```python
from build123d import *

# Parameters (mm, degrees)
F0_W     = 40
F0_H     = 10
F1_DEPTH = 5
F2_DEPTH = 92
F3_DEPTH = 50


with BuildPart() as f1:
    # F0 (on Top) → F1 (new body)
    with BuildSketch(Plane.XY):
        with Locations((-1.222661, 7.045219)):
            Rectangle(F0_W, F0_H)
    extrude(amount=F1_DEPTH)

    # F0 (on Top) → F2 (join)
    with BuildSketch(Plane.XY):
        Polygon((-26.222661, 12.045219), (-21.222661, 12.045219), (18.777339, 12.045219), (23.777339, 12.045219), (23.777339, 17.045219), (-26.222661, 17.045219), align=None)
    extrude(amount=F2_DEPTH)

    # F0 (on Top) → F3 (join)
    with BuildSketch(Plane.XY):
        Polygon((-21.222661, 2.045219), (-21.222661, 12.045219), (-26.222661, 12.045219), (-26.222661, -2.954781), (23.777339, -2.954781), (23.777339, 12.045219), (18.777339, 12.045219), (18.777339, 2.045219), align=None)
    extrude(amount=F3_DEPTH)


solid = f1.part
```
Build history of the part. All positions in model axes, mm. A direction names the side the tool comes from. Round coordinates to 2 decimals unless told otherwise and drop trailing zeros. Write each loop counter-clockwise with the first axis right and the second up, starting at its lowest first coordinate (ties: lowest second). Pieces come first, ordered by that corner, then holes.
1) Band-saw the part on C-C, the plane y = 4.5. List the corners of the cut face in (x, z).
2) 3-axis set-ups, long thin cutter, end or side, ignore diameter. For faces 4 (the flat face through (-21.223, 7, 27)), 5 (the flat face through (-26.223, 9, 35)), 6 (the flat face through (-2, 1, 50)): which of +Z, -Z, +X, -X, +Y, -Y reach the whole face in a straight line?
3) Mould opens along Y. For faces 1 (the flat face through (-2, 12.045, 48)), 2 (the flat face through (-2, 7, 0)), 3 (the flat face through (-2, -2.955, 25)) say: +Y half, -Y half, draft (parallel to the pull), parting line (faces both ways), or undercut.
4) Band-saw the part on D-D, the plane z = 55. List the corners of the cut face in (x, y).
5) Band-saw the part on B-B, the plane x = -4. List the corners of the cut face in (y, z), and give its area (3 significant figures).
6) Pin check, flat tips, straight feed: pin 1 (7.5 mm diameter, centred on x = 0, y = 6.5, fed in from +Z); pin 2 (11 mm diameter, centred on x = -9, y = 6.5, fed in from +Z); pin 3 (25 mm diameter, centred on x = 9, z = 67, fed in from -Y). Stop position of each tip, or through.
7) Drill centre lines: probe 1 along Y at (x, z) = (2, 39); probe 2 along X at (y, z) = (10.5, 45); probe 3 along Z at (x, y) = (-19, 9.5). Where is each one in solid material? Low to high.
8) Band-saw the part on A-A, the plane z = 16. List the corners of the cut face in (x, y), and give its area (3 significant figures).
Ans:
1. outline: (-26.22, 0) - (23.78, 0) - (23.78, 50) - (18.78, 50) - (18.78, 5) - (-21.22, 5) - (-21.22, 50) - (-26.22, 50) - close
2. face 4: +Z
2. face 5: +Z, -Z, -X, +Y, -Y
2. face 6: +Z, +X, -X, -Y
3. face 1: undercut
3. face 2: draft
3. face 3: -Y half
4. outline: (-26.22, 12.05) - (23.78, 12.05) - (23.78, 17.05) - (-26.22, 17.05) - close
5. outline: (-2.95, 0) - (17.05, 0) - (17.05, 92) - (12.05, 92) - (12.05, 5) - (2.05, 5) - (2.05, 50) - (-2.95, 50) - close
5. area: 760 mm2
6. pin 1: stops at z = 5
6. pin 2: stops at z = 50
6. pin 3: stops at y = 12.05
7. probe 1: y = -2.95 to 2.05, 12.05 to 17.05
7. probe 2: x = -26.22 to -21.22, 18.78 to 23.78
7. probe 3: z = 0 to 5
8. outline: (-26.22, -2.95) - (23.78, -2.95) - (23.78, 17.05) - (-26.22, 17.05) - close; hole (-21.22, 2.05) - (18.78, 2.05) - (18.78, 12.05) - (-21.22, 12.05) - close
8. area: 600 mm2
